```python
from build123d import *

# Parameters (mm, degrees)
F0_R     = 9.525
F1_DEPTH = 9.525
F2_R     = 9.525
F3_DEPTH = 19.05


# Not quite as in the source:
# - a feature of the source that left no trace in its solid (it failed there, or was rolled back) is left out
# - a pattern or mirror of a feature is missing from the dataset's text; its kind, count and spacing are read off the source's solid


with BuildPart() as f1:
    # F0 (on Front) → F1 (new body, symmetric)
    with BuildSketch(Plane.XZ):
        with BuildLine():
            ThreePointArc((76.2, -15.875), (92.075, 0), (76.2, 15.875))
            Line((76.2, 15.875), (-76.2, 15.875))
            ThreePointArc((-76.2, 15.875), (-92.075, 0), (-76.2, -15.875))
            Line((-76.2, -15.875), (76.2, -15.875))
        make_face()
        with Locations((-76.2, 0)):
            Circle(F0_R, mode=Mode.SUBTRACT)
        with Locations((76.2, 0)):
            Circle(F0_R, mode=Mode.SUBTRACT)
        with Locations((76.2, 0)):
            Circle(F0_R)
    extrude(amount=F1_DEPTH, both=True)

    # F2 (on face) → F3 (join)
    with BuildSketch(Plane.XZ.offset(9.525)):
        Circle(F2_R)
    f3 = extrude(amount=F3_DEPTH)

    # F3_copies: F3 across plane
    add(f3.mirror(Plane(origin=(38.1, 0, 0), x_dir=(0, 0, 1), z_dir=(1, 0, 0))))


solid = f1.part
```
Work out the finished part from the listing and answer in its coordinate system (mm). A direction names the side the tool comes from. Coordinates: 2 decimals unless noted, no trailing zeros. Loops run counter-clockwise (first coordinate to the right, second up) from the corner with the lowest first, then second, coordinate; pieces in that order, holes last.
1) For faces 5 (the cylindrical face through (92.07, -0.13, -0.35)), 6 (the cylindrical face through (-7.559, -18.917, -5.796)), determine the directions among +Z, -Z, +X, -X, +Y, -Y from which every point of the face is accessible in a straight line to the end or side of a thin tool.
Results:
face 5: +X, +Y, -Y
face 6: -Y
2) Section D-D (y = 4) is taken. Give the vertices of the cut face in (x, z) (3 decimals), plus the area to 3 significant figures.
Results:
outline: (-76.2, -15.875) - (76.2, -15.875) arc R15.875 ccw to (76.2, 15.875) - (-76.2, 15.875) arc R15.875 ccw to start; hole circle Ø19.05 at (-76.2, 0)
area: 5,350 mm2
3) Flat-ended cylindrical pins translate along their axes: pin 1 (12 mm diameter, centred on y = -17.5, z = -8.5, fed in from +X); pin 2 (5 mm diameter, centred on x = 9, z = -8.5, fed in from -Y) (3 decimals); pin 3 (8 mm diameter, centred on y = -6.5, z = 4, fed in from -X) (3 decimals); pin 4 (1 mm diameter, centred on y = -3.5, z = -8, fed in from -X). Find the tip coordinate at first contact, or state that the pin passes through.
Results:
pin 1: stops at x = 85.39
pin 2: stops at y = -9.525
pin 3: stops at x = -92.075
pin 4: stops at x = -90.19
4) Section A-A (z = 0) is taken. Give the vertices of the cut face in (x, y) (3 decimals).
Results:
outline: (-92.075, -9.525) - (-85.725, -9.525) - (-85.725, 9.525) - (-92.075, 9.525) - close; (-66.675, -9.525) - (-9.525, -9.525) - (-9.525, -28.575) - (9.525, -28.575) - (9.525, -9.525) - (66.675, -9.525) - (66.675, -28.575) - (85.725, -28.575) - (85.725, -9.525) - (92.075, -9.525) - (92.075, 9.525) - (-66.675, 9.525) - close
5) Section B-B (x = 0) is taken. Give the vertices of the cut face in (y, z) (3 decimals), plus the area to 3 significant figures.
Results:
outline: (-28.575, -9.525) - (-9.525, -9.525) - (-9.525, -15.875) - (9.525, -15.875) - (9.525, 15.875) - (-9.525, 15.875) - (-9.525, 9.525) - (-28.575, 9.525) - close
area: 968 mm2
6) Section C-C (y = -20.5) is taken. Give the vertices of the cut face in (x, z) (3 decimals).
Results:
outline: circle Ø19.05 at (0, 0); circle Ø19.05 at (76.2, 0)
7) For a pull along X with two mould halves and no side action, classify faces 1 (the flat face through (-1, 0, -15.875)), 2 (the flat face through (-1, -9.525, -10)), 3 (the cylindrical face through (85.716, -18.917, 0.419)), 4 (the cylindrical face through (-92.07, -0.13, 0.35)) as +X half, -X half, draft (parallel to the pull), parting line (faces both ways), or undercut.
Results:
face 1: draft
face 2: undercut
face 3: undercut
face 4: -X half
8) Consider probe 1 along Z at (x, y) = (-76.2, -5.5) (3 decimals); probe 2 along Y at (x, z) = (-54, -6) (3 decimals); probe 3 along X at (y, z) = (-6, -3). Determine where each line is inside the solid, lowest interval first.
Results:
probe 1: z = -15.875 to -9.525, 9.525 to 15.875
probe 2: y = -9.525 to 9.525
probe 3: x = -91.79 to -85.24, -67.16 to 91.79
